Check sheet for the drawn part. Datum: minimum x, y, z corner. Units: mm. Give positions to 0.01 mm unless a question says otherwise; leave off trailing zeros. Write each loop counter-clockwise with the first axis right and the second up, starting at its lowest first coordinate (ties: lowest second). Pieces come first, ordered by that corner, then holes. Notation, with made-up numbers: (-13, 83.5) - (18, 83.5) arc R26 cw to (18, 122.5) - close; hole circle Ø1 at (-12, 79.5). An arc over 180 degrees is marked (long way). Use a Markdown table: item, result.
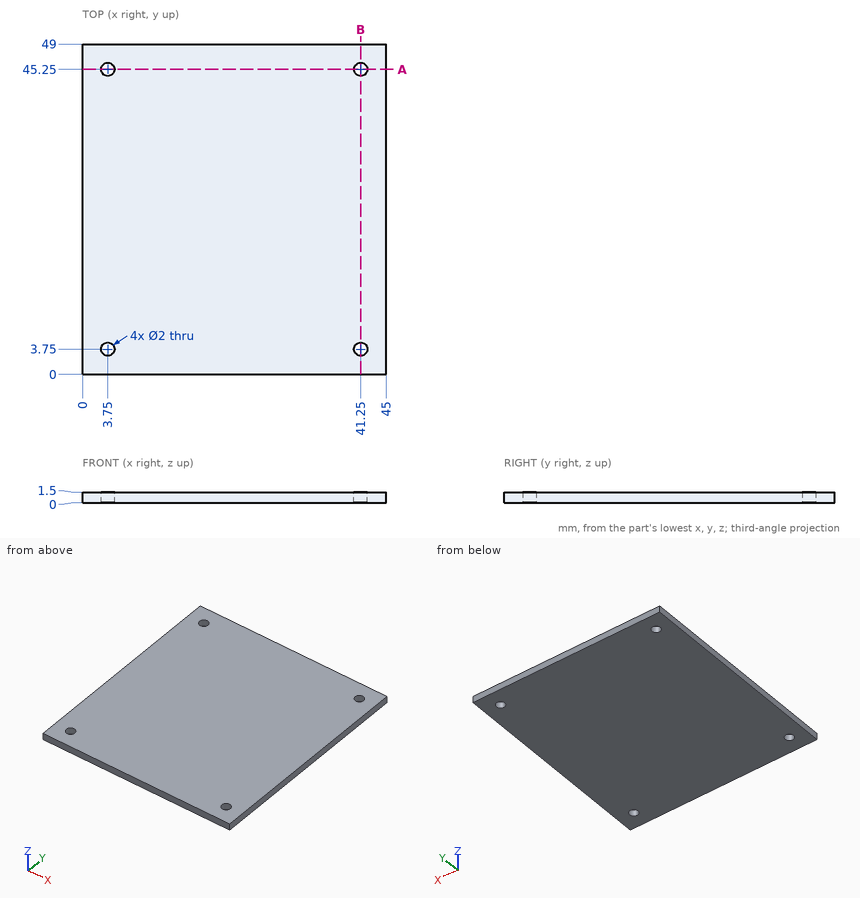
1) Material ranges on L1, parallel to Y at x = 3.75, z = 0.95; L2, parallel to X at y = 45.25, z = 1.2; L3, parallel to Y at x = 4.5, z = 0.75, recorded low to high. Write a range as from..to.
Working result:
| item | result |
|---|---|
| L1 | y = 0..2.75, 4.75..44.25, 46.25..49 |
| L2 | x = 0..2.75, 4.75..40.25, 42.25..45 |
| L3 | y = 0..3.09, 4.41..44.59, 45.91..49 |
2) Depth check by flat-ended pin: P1, Ø1.2, axis at x = 3.75, y = 45.25, coming from the -Z side. Enter the tip coordinate at first touch or a pass-through.
Working result:
| item | result |
|---|---|
| P1 | passes through |
3) Section check A-A on y = 45.25. Record the boundary of the cut face in (x, z).
Working result:
| item | result |
|---|---|
| outline | (0, 0) - (2.75, 0) - (2.75, 1.5) - (0, 1.5) - close; (4.75, 0) - (40.25, 0) - (40.25, 1.5) - (4.75, 1.5) - close; (42.25, 0) - (45, 0) - (45, 1.5) - (42.25, 1.5) - close |
4) Section check B-B on x = 41.25. Record the boundary of the cut face in (y, z).
Working result:
| item | result |
|---|---|
| outline | (0, 0) - (2.75, 0) - (2.75, 1.5) - (0, 1.5) - close; (4.75, 0) - (44.25, 0) - (44.25, 1.5) - (4.75, 1.5) - close; (46.25, 0) - (49, 0) - (49, 1.5) - (46.25, 1.5) - close |
